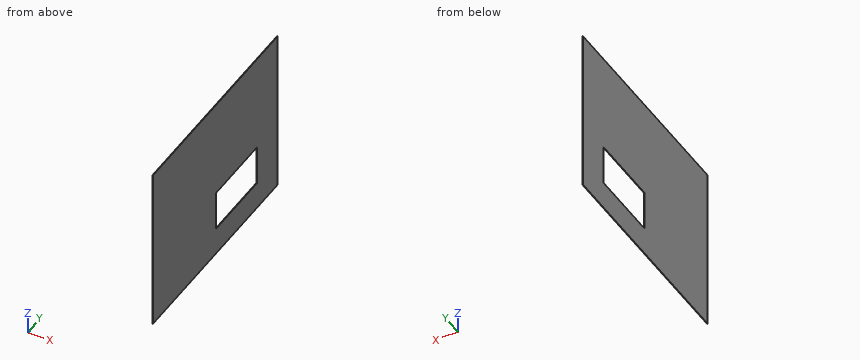
```python
from build123d import *

# Parameters (mm, degrees)
SKETCH1_W            = 914.4
SKETCH1_H            = 1219.2
PLATE_BASE_DEPTH     = 1.5875
TANK_HOLE_DEPTH      = 763.001653644
TANK_HOLE_DEPTH_BACK = 763.001653644
SKETCH4_W            = 220
SKETCH4_H            = 400


with BuildPart() as part:
    # Sketch1 → Plate_Base (new, symmetric)
    with BuildSketch(Plane(origin=(0, 0, 0), x_dir=(0, 0, -1), z_dir=(1, 0, 0))):
        Rectangle(SKETCH1_W, SKETCH1_H)
    extrude(amount=PLATE_BASE_DEPTH, both=True)

    # Sketch4 → Tank_Hole (cut, two sides: drawn at the far end of the back side and taken through both)
    with BuildSketch(Plane(origin=(0, 0, 0), x_dir=(0, 0, -1), z_dir=(1, 0, 0)).offset(-TANK_HOLE_DEPTH_BACK)):
        with Locations((194.8, 206.4)):
            Rectangle(SKETCH4_W, SKETCH4_H)
    extrude(amount=TANK_HOLE_DEPTH + TANK_HOLE_DEPTH_BACK, mode=Mode.SUBTRACT)


solid = part.part
```
Could you check a few things on this model? Use its own coordinates, in mm. Round coordinates to 2 decimals unless told otherwise and drop trailing zeros. Order: outer loops, then holes, each group sorted by start corner. A loop starts at its lowest first (then second) coordinate and runs counter-clockwise, first axis right, second up. Notation, with made-up numbers: M 77.25,-39.5 L 91.25,-39.5 A22 ccw 91.25,-16.5 Z; hole C 51,-14 d7. An arc over 180 degrees is marked long. One line per question, with ' | ' between items. Start each with the question number.
(1) Suppose I cut it at B-B on y = 137. List the corners of the cut face in (x, z) for me, then the cut area to 3 significant figures.
(2) Suppose I cut it at C-C on z = -277.5. List the corners of the cut face in (x, y) for me.
(3) Please list where these lines run through material, in increasing order: line 1 along Y through (x, z) = (1, -279.5); line 2 along Z through (x, y) = (1.3, 284.5).
(4) Suppose I cut it at A-A on x = 0.05. List the corners of the cut face in (y, z) for me, then the cut area to 3 significant figures.
Geometry results:
1) outline: M -1.59,-457.2 L 1.59,-457.2 L 1.59,-304.8 L -1.59,-304.8 Z; M -1.59,-84.8 L 1.59,-84.8 L 1.59,457.2 L -1.59,457.2 Z | area: 2,200 mm²
2) outline: M -1.59,-609.6 L 1.59,-609.6 L 1.59,6.4 L -1.59,6.4 Z; M -1.59,406.4 L 1.59,406.4 L 1.59,609.6 L -1.59,609.6 Z
3) line 1: -609.6 to 6.4, 406.4 to 609.6 | line 2: -457.2 to -304.8, -84.8 to 457.2
4) outline: M -609.6,-457.2 L 609.6,-457.2 L 609.6,457.2 L -609.6,457.2 Z; hole M 6.4,-304.8 L 406.4,-304.8 L 406.4,-84.8 L 6.4,-84.8 Z | area: 1,030,000 mm²
